from build123d import *

# Parameters (mm, degrees)
SKETCH_1_W             = 20
SKETCH_1_H             = 28.9
EXTRUDE_1_DEPTH        = 8
SKETCH_2_W             = 3.5
SKETCH_2_H             = 9
CUT_EXTRUDE_1_DEPTH    = 32.610283137
HOLE_WIZARD_M3_1_D     = 2.5
HOLE_WIZARD_M3_1_DEPTH = 6.5
HOLE_WIZARD_M3_1_TIP   = 0.751075774


with BuildPart() as part:
    # 草图1 → 凸台-拉伸1 (new body)
    with BuildSketch(Plane(origin=(0, 0, 0), x_dir=(0, 0, -1), z_dir=(1, 0, 0))):
        Rectangle(SKETCH_1_W, SKETCH_1_H)
    extrude(amount=EXTRUDE_1_DEPTH)

    # 草图2 → 切除-拉伸1 (cut, through all)
    with BuildSketch(Plane(origin=(0, 14.45, 0), x_dir=(1, 0, 0), z_dir=(0, 1, 0))):
        with Locations((1.75, 0)):
            Rectangle(SKETCH_2_W, SKETCH_2_H)
    extrude(amount=-CUT_EXTRUDE_1_DEPTH, mode=Mode.SUBTRACT)

    # M3 螺纹孔1
    with Locations(Plane(origin=(8, 0, 0), x_dir=(0, 0, -1), z_dir=(1, 0, 0))):
        with Locations((-7.5, 5), (7.5, -5), (-7.5, -5), (7.5, 5)):
            Hole(HOLE_WIZARD_M3_1_D / 2, depth=HOLE_WIZARD_M3_1_DEPTH)
            with Locations((0, 0, -(HOLE_WIZARD_M3_1_DEPTH + HOLE_WIZARD_M3_1_TIP / 2))):  # 118° drill point
                Cone(0, HOLE_WIZARD_M3_1_D / 2, HOLE_WIZARD_M3_1_TIP, mode=Mode.SUBTRACT)


solid = part.part
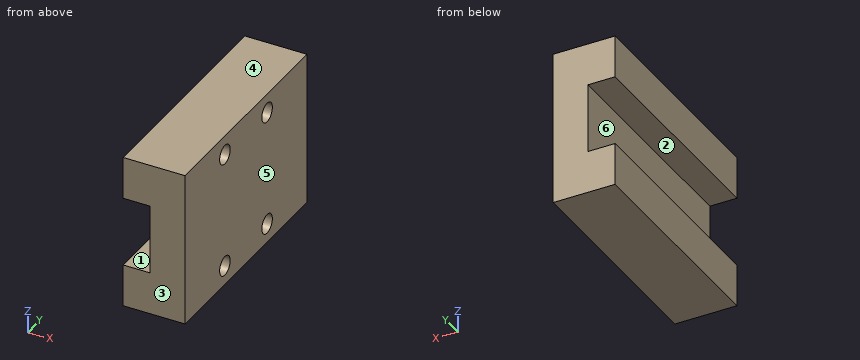
Work out the finished part from the listing and answer in its coordinate system (mm). Face numbers are marked on the shaded views. A direction names the side the tool comes from. Coordinates: 2 decimals unless noted, no trailing zeros. Write each loop counter-clockwise with the first axis right and the second up, starting at its lowest first coordinate (ties: lowest second). Pieces come first, ordered by that corner, then holes. Notation, with made-up numbers: M -5.75,-26 L 13.25,-26 A25 ccw 13.25,10 Z; hole C 19,-9.75 d10. An arc over 180 degrees is marked long. Use one line per item in the form item = value. Start each with the question number.
1. The mould has two halves that part along Z. Classify the marked faces 1, 2, 3 and 4: released by +Z, released by -Z, zero draft, split by the parting line, or undercut.
2. Each of these flat-tipped pins is pushed along its axis until it touches: P1, Ø7, axis at y = 1, z = 0, coming from the -X side; P2, Ø2, axis at y = -5, z = 7.5, coming from the +X side. Where does it stop, or does it pass through?
3. The part is cut by section C-C (z = 4). Give the vertices of the cut face in (x, y).
4. The part is cut by section B-B (y = 8). Give the vertices of the cut face in (x, z), plus the area to 4 significant figures.
5. Straight lines are drawn through the part: probe 1 along Y at (x, z) = (2, -7.5); probe 2 along Z at (x, y) = (5.75, -5); probe 3 along Z at (x, y) = (3, -5). For each, find the intervals that lie inside material, in ascending order. Write a range as from..to.
6. A tool of negligible diameter and unlimited length cuts with its end or side. For the marked faces 5 and 6, from which of +Z, -Z, +X, -X, +Y, -Y can it reach the whole face along a straight path? Write none if from no direction.
7. The part is cut by section A-A (x = 2). Give the vertices of the cut face in (y, z).
Evaluation:
q1.face_1 = undercut
q1.face_2 = undercut
q1.face_3 = zero draft
q1.face_4 = released by +Z
q2.P1 = 3.5
q2.P2 = 1.35
q3.outline = M 3.5,-14.45 L 8,-14.45 L 8,14.45 L 3.5,14.45 Z
q4.outline = M 0,-10 L 8,-10 L 8,10 L 0,10 L 0,4.5 L 3.5,4.5 L 3.5,-4.5 L 0,-4.5 Z
q4.area = 128.5 mm^2
q5.probe_1 = -14.45..-6.25, -3.75..3.75, 6.25..14.45
q5.probe_2 = -10..-8.75, -6.25..6.25, 8.75..10
q5.probe_3 = -10..-8.75, -6.25..-4.5, 4.5..6.25, 8.75..10
q6.face_5 = +Z, -Z, +X, +Y, -Y
q6.face_6 = -X, +Y, -Y
q7.outline = M -14.45,-10 L 14.45,-10 L 14.45,-4.5 L -14.45,-4.5 Z; M -14.45,4.5 L 14.45,4.5 L 14.45,10 L -14.45,10 Z; hole C -5,-7.5 d2.5; hole C -5,7.5 d2.5; hole C 5,-7.5 d2.5; hole C 5,7.5 d2.5
